Read the model definition and answer for the solid it produces. Units are mm, in the model's axes. A direction names the side the tool comes from. Round coordinates to 2 decimals unless told otherwise and drop trailing zeros. Write each loop counter-clockwise with the first axis right and the second up, starting at its lowest first coordinate (ties: lowest second). Pieces come first, ordered by that corner, then holes. Notation, with made-up numbers: (48, 76.5) - (66, 76.5) arc R27 ccw to (66, 107.5) - close; hole circle Ø7 at (-29, -4). An arc over 180 degrees is marked (long way). Answer as CSV lines item,"result". Start each with the question number.
1) For a pull along Z with two mould halves and no side action, classify faces 6 (the flat face through (-6.54, 59.79, -17.35)), 7 (the flat face through (-57, 60, -26)), 8 (the cylindrical face through (-90, 70, 0)) as +Z half, -Z half, draft (parallel to the pull), parting line (faces both ways), or undercut.
2) Find section D-D on y = 43. Determine the outline of the cut face in (x, z), then the cut area to 3 significant figures.
3) Find section C-C on z = 0. Determine the outline of the cut face in (x, y), then the cut area to 3 significant figures.
4) Which of the six approach directions +Z, -Z, +X, -X, +Y, -Y give full straight-line access (tool end or side, diameter ignored) to faces 1 (the flat face through (-76, 65, 0)), 2 (the flat face through (-35, 60, -30)), 3 (the flat face through (-6.727, 59.79, 17.67)), 4 (the flat face through (-83, 55, -21)), 5 (the flat face through (-57, 60, 25))?
5) Each of these flat-tipped pins is pushed along its axis until it touches: pin 1 (1.5 mm diameter, centred on x = -93, y = 28, fed in from +Z); pin 2 (8 mm diameter, centred on y = 44, z = -13.5, fed in from -X); pin 3 (2.5 mm diameter, centred on y = 67, z = 26.5, fed in from -X); pin 4 (11 mm diameter, centred on y = 38.5, z = 27.5, fed in from +X). Where does it stop, or does it pass through?
6) Find section B-B on y = 69. State how many separate pieces and enclosed holes the cut face has, then the cut area to 3 significant figures.
7) Consider line 1 along Z through (x, y) = (-35, 52); line 2 along Y through (x, z) = (-46, 20); line 3 along Z through (x, y) = (-88, 36.5). Determine where each line is inside the solid, lowest interval first.
8) Find section A-A on x = -35. Determine the outline of the cut face in (y, z), then the cut area to 3 significant figures.
from build123d import *

# Parameters (mm, degrees)
BOSS_EXTRUDE2_DEPTH = 75
CUT_EXTRUDE1_DEPTH  = 50
CUT_EXTRUDE2_DEPTH  = 10
SKETCH7_R           = 5
CUT_EXTRUDE3_DEPTH  = 10
SKETCH8_R           = 7.5
CUT_EXTRUDE4_DEPTH  = 153.707924315


with BuildPart() as part:
    # Sketch3 → Boss-Extrude2 (new body)
    with BuildSketch(Plane(origin=(0, 0, 0), x_dir=(1, 0, 0), z_dir=(0, 1, 0))):
        with BuildLine():
            Line((0, -6.019237886), (0, 6.019237886))
            Line((0, 6.019237886), (-13.267949192, 29))
            ThreePointArc((-13.267949192, 29), (-14, 29.732050808), (-15, 30))
            Line((-15, 30), (-55, 30))
            ThreePointArc((-55, 30), (-56.414213562, 29.414213562), (-57, 28))
            Line((-57, 28), (-57, 23))
            ThreePointArc((-57, 23), (-57.585786438, 21.585786438), (-59, 21))
            Line((-59, 21), (-98, 21))
            ThreePointArc((-98, 21), (-99.414213562, 21.585786438), (-100, 23))
            Line((-100, 23), (-100, 33))
            ThreePointArc((-100, 33), (-100.585786438, 34.414213562), (-102, 35))
            Line((-102, 35), (-117, 35))
            ThreePointArc((-117, 35), (-117.975900073, 34.745743122), (-118.70367084, 34.047619048))
            ThreePointArc((-118.70367084, 34.047619048), (-128.33436854, 0), (-118.70367084, -34.047619048))
            ThreePointArc((-118.70367084, -34.047619048), (-117.975900073, -34.745743122), (-117, -35))
            Line((-117, -35), (-102, -35))
            ThreePointArc((-102, -35), (-100.585786438, -34.414213562), (-100, -33))
            Line((-100, -33), (-100, -23))
            ThreePointArc((-100, -23), (-99.414213562, -21.585786438), (-98, -21))
            Line((-98, -21), (-59, -21))
            ThreePointArc((-59, -21), (-57.585786438, -21.585786438), (-57, -23))
            Line((-57, -23), (-57, -28))
            ThreePointArc((-57, -28), (-56.414213562, -29.414213562), (-55, -30))
            Line((-55, -30), (-15, -30))
            ThreePointArc((-15, -30), (-14, -29.732050808), (-13.267949192, -29))
            Line((-13.267949192, -29), (0, -6.019237886))
        make_face()
    extrude(amount=BOSS_EXTRUDE2_DEPTH)

    # Sketch4 → Cut-Extrude1 (cut, symmetric)
    with BuildSketch(Plane.XY):
        Polygon((0, 45), (-75, 45), (-128.33436854, 0), (0, 0), align=None)
    extrude(amount=CUT_EXTRUDE1_DEPTH, both=True, mode=Mode.SUBTRACT)

    # Sketch5 → Cut-Revolve1 (revolve, cut)
    with BuildSketch(Plane.XY, mode=Mode.PRIVATE) as cut_revolve1_sk:
        Polygon((-35, 75), (-50, 75), (-44.226497308, 65), (-44.226497308, 57.990381057), (-42.5, 55), (-42.5, 45), (-35, 45), align=None)
    revolve(cut_revolve1_sk.sketch.rotate(Axis((-35, 75, 0), (0, -1, 0)), 270), axis=Axis((-35, 75, 0), (0, -1, 0)), mode=Mode.SUBTRACT)

    # Sketch6 → Cut-Extrude2 (cut)
    with BuildSketch(Plane(origin=(0, 75, 0), x_dir=(1, 0, 0), z_dir=(0, 1, 0))):
        with BuildLine():
            Line((-55.908593, 42.121600501), (-57.789518761, 68.995445657))
            ThreePointArc((-57.789518761, 68.995445657), (-88.91346012, 13.942618456), (-76.134860141, -47.994615024))
            Line((-76.134860141, -47.994615024), (-58.539070897, -38.381990289))
            ThreePointArc((-58.539070897, -38.381990289), (-69.962661294, 2.286050005), (-55.908593, 42.121600501))
        make_face()
    extrude(amount=-CUT_EXTRUDE2_DEPTH, mode=Mode.SUBTRACT)

    # Sketch7 → Cut-Extrude3 (cut)
    with BuildSketch(Plane(origin=(0, 65, 0), x_dir=(1, 0, 0), z_dir=(0, 1, 0))):
        with Locations(Location((-79.033128747, 15, 0), (0, 0, 270))):
            Circle(SKETCH7_R)
        with Locations(Location((-83, 0, 0), (0, 0, 270))):
            Circle(SKETCH7_R)
        with Locations(Location((-79.033128747, -15, 0), (0, 0, 270))):
            Circle(SKETCH7_R)
    extrude(amount=-CUT_EXTRUDE3_DEPTH, mode=Mode.SUBTRACT)

    # Sketch8 → Cut-Extrude4 (cut, through all)
    with BuildSketch(Plane(origin=(0, 0, 0), x_dir=(0, 0, -1), z_dir=(1, 0, 0))):
        with Locations(Location((0, 25, 0), (0, 0, 90))):
            Circle(SKETCH8_R)
    extrude(amount=-CUT_EXTRUDE4_DEPTH, mode=Mode.SUBTRACT)


solid = part.part
Check values:
1,face 6,"-Z half"
1,face 7,"draft"
1,face 8,"undercut"
2,outline,"(-118.7, -34.05) arc R2 ccw to (-117, -35) - (-102, -35) arc R2 ccw to (-100, -33) - (-100, -23) arc R2 cw to (-98, -21) - (-77.37, -21) - (-77.37, 21) - (-98, 21) arc R2 cw to (-100, 23) - (-100, 33) arc R2 ccw to (-102, 35) - (-117, 35) arc R2 ccw to (-118.7, 34.05) arc R65 ccw to start"
2,area,"2,700 mm^2"
3,outline,"(-128.33, 0) - (-107.59, 17.5) - (-128.33, 17.5) - close; (-128.33, 32.5) - (-89.82, 32.5) - (-75, 45) - (-42.5, 45) - (-42.5, 55) - (-44.23, 57.99) - (-44.23, 65) - (-50, 75) - (-70, 75) - (-70, 65) - (-78, 65) - (-78, 55) - (-88, 55) - (-88, 65) - (-90, 65) - (-90, 75) - (-128.33, 75) - close; (-27.5, 45) - (0, 45) - (0, 75) - (-20, 75) - (-25.77, 65) - (-25.77, 57.99) - (-27.5, 55) - close"
3,area,"3,730 mm^2"
4,face 1,"+Y"
4,face 2,"-Z, +X, +Y, -Y"
4,face 3,"+Z, +X, +Y, -Y"
4,face 4,"-Z, +Y, -Y"
4,face 5,"+Z, +Y, -Y"
5,pin 1,"passes through"
5,pin 2,"stops at x = -127.64"
5,pin 3,"stops at x = -123.23"
5,pin 4,"stops at x = -99.73"
6,separate pieces,"2"
6,enclosed holes,"1"
6,area,"5,380 mm^2"
7,line 1,"z = -30 to -7.5, 7.5 to 30"
7,line 2,"y = 45 to 75"
7,line 3,"z = -21 to 21"
8,outline,"(45, -30) - (75, -30) - (75, -15) - (65, -9.23) - (57.99, -9.23) - (55, -7.5) - (45, -7.5) - close; (45, 7.5) - (55, 7.5) - (57.99, 9.23) - (65, 9.23) - (75, 15) - (75, 30) - (45, 30) - close"
8,area,"1,230 mm^2"
